Answer from the drawing. Dimensions are ordinates in mm from the lowest x, y and z of the part. Coordinates: 2 decimals unless noted, no trailing zeros. Loops run counter-clockwise (first coordinate to the right, second up) from the corner with the lowest first, then second, coordinate; pieces in that order, holes last. Notation, with made-up numbers: (20, 6.5) - (56, 6.5) arc R12 ccw to (56, 23.5) - close; hole circle Ø3 at (-32, -0.5). An arc over 180 degrees is marked (long way). Write each question's results on one line, items separated by ' | '. Start each with the question number.
1. This flat-tipped pin is pushed along its axis until it touches: P1, Ø12, axis at x = 12.5, z = 81, coming from the -Y side. Where does it stop, or does it pass through?
2. Determine the mould class of the marked faces 1, 2, 3 and 4 for opening direction X: released by +X, released by -X, zero draft, split by the parting line, or undercut.
3. A cutting plane is placed at D-D on x = 33. Determine the outline of the cut face in (y, z), then the cut area to 3 significant figures.
4. A cutting plane is placed at B-B on x = 16.5. Determine the outline of the cut face in (y, z).
5. A cutting plane is placed at A-A on y = 20.5. Determine the outline of the cut face in (x, z) (1 decimal), then the cut area to 3 significant figures.
6. Find the intervals of material crossed by line 1 along Y through (x, z) = (17.5, 86.5) (1 decimal); line 2 along Y through (x, z) = (20.5, 81); line 3 along X through (y, z) = (19, 64) (1 decimal), in increasing order. Write a range as [from, to].
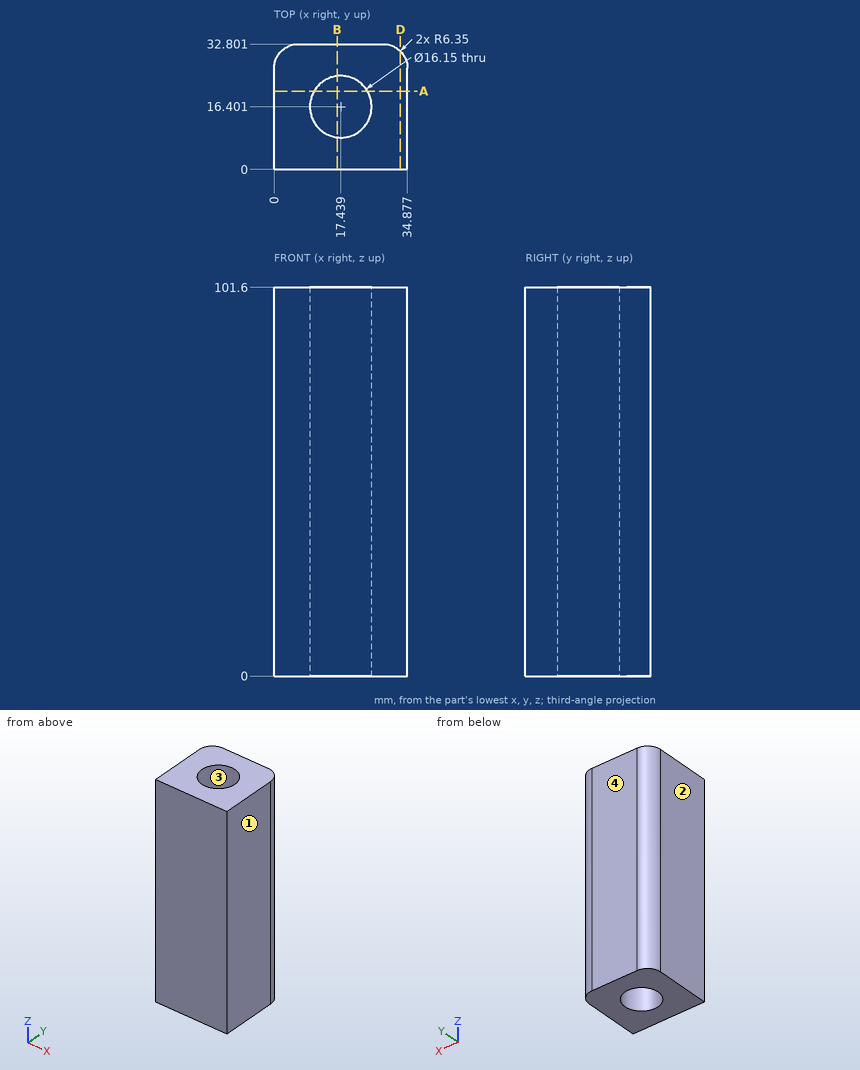
Values:
1) P1: y = 0
2) face 1: released by +X | face 2: released by -X | face 3: undercut | face 4: zero draft
3) outline: (0, 0) - (30.96, 0) - (30.96, 101.6) - (0, 101.6) - close | area: 3,150 mm^2
4) outline: (0, 0) - (8.38, 0) - (8.38, 101.6) - (0, 101.6) - close; (24.42, 0) - (32.8, 0) - (32.8, 101.6) - (24.42, 101.6) - close
5) outline: (0, 0) - (10.5, 0) - (10.5, 101.6) - (0, 101.6) - close; (24.4, 0) - (34.9, 0) - (34.9, 101.6) - (24.4, 101.6) - close | area: 2,130 mm^2
6) line 1: [0, 8.3], [24.5, 32.8] | line 2: [0, 8.93], [23.87, 32.8] | line 3: [0, 9.8], [25.1, 34.9]
